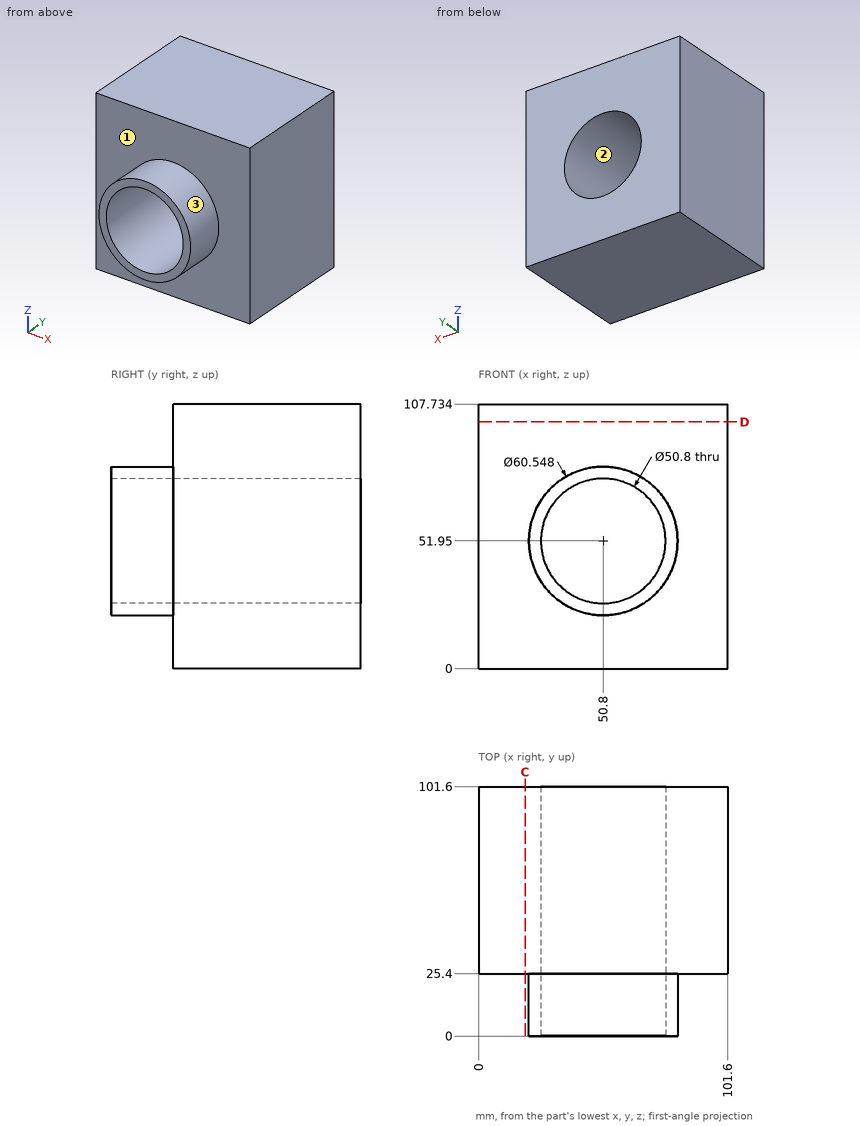
Here's the drawing with two shaded views (mm, measured from the low corner). I have some questions. Give positions to 0.01 mm unless a question says otherwise; leave off trailing zeros. Order: outer loops, then holes, each group sorted by start corner. A loop starts at its lowest first (then second) coordinate and runs counter-clockwise, first axis right, second up. Notation, with made-up numbers: (58.25, 35) - (103.25, 35) arc R17 cw to (103.25, 43) - close; hole circle Ø3 at (20, 87.5). An arc over 180 degrees is marked (long way). Use a Markdown table: item, result. Add a question column.
Q1. If we mould it in two halves opening along Z, with no side actions, what happens to the marked faces 1, 2 and 3? For each: released by +Z, released by -Z, zero draft, split by the parting line, or undercut.
Q2. Please list where these lines run through material, in increasing order: line 1 along Z through (x, y) = (50, 43) (1 decimal); line 2 along Y through (x, z) = (6, 98); line 3 along X through (y, z) = (54.5, 43).
Q3. If we section it at C-C on x = 19: Write out the boundary of the cut face in (y, z) (1 decimal), plus the area to 3 significant figures.
Q4. I'm going to push flat-ended pins straight in: pin 1 (2 mm diameter, centred on y = 21, z = 28, fed in from -X) (1 decimal); pin 2 (2 mm diameter, centred on y = 39, z = 33, fed in from -X). Where does each tip first touch, or does it pass through?
Q5. If we section it at D-D on z = 100.5: Write out the boundary of the cut face in (x, y).
Answers follow:
| question | item | result |
|---|---|---|
| 1 | face 1 | zero draft |
| 1 | face 2 | undercut |
| 1 | face 3 | split by the parting line |
| 2 | line 1 | z = 0 to 26.6, 77.3 to 107.7 |
| 2 | line 2 | y = 25.4 to 101.6 |
| 2 | line 3 | x = 0 to 27.03, 74.57 to 101.6 |
| 3 | outline | (25.4, 0) - (101.6, 0) - (101.6, 107.7) - (25.4, 107.7) - close |
| 3 | area | 8,210 mm^2 |
| 4 | pin 1 | stops at x = 31.1 |
| 4 | pin 2 | stops at x = 0 |
| 5 | outline | (0, 25.4) - (101.6, 25.4) - (101.6, 101.6) - (0, 101.6) - close |
